Answer from the drawing. Dimensions are ordinates in mm from the lowest x, y and z of the part. A direction names the side the tool comes from. Coordinates: 2 decimals unless noted, no trailing zeros. Order: outer loops, then holes, each group sorted by start corner. A loop starts at its lowest first (then second) coordinate and runs counter-clockwise, first axis right, second up.
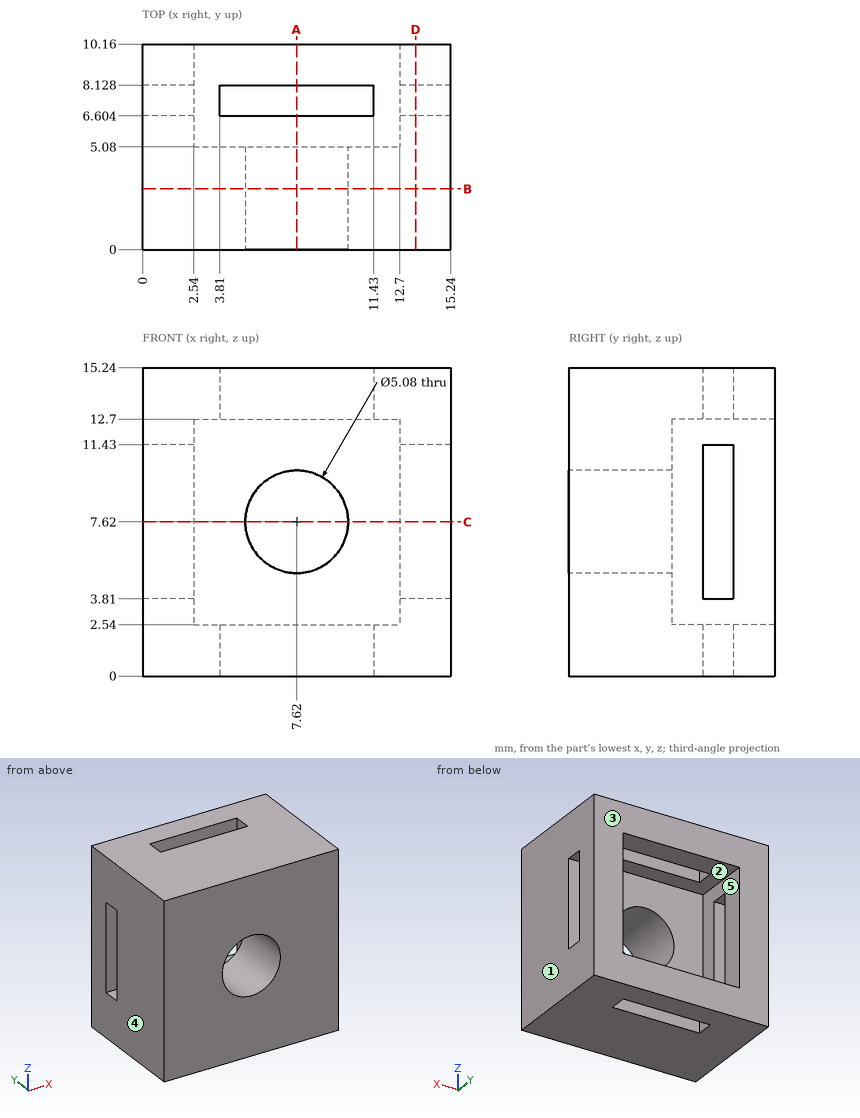
1) Section B-B (y = 3) is taken. Give the vertices of the cut face in (x, z), then the cut area to 3 significant figures.
2) Determine the mould class of the marked faces 1, 2 and 3 for opening direction X: released by +X, released by -X, zero draft, split by the parting line, or undercut.
3) Section A-A (x = 7.62) is taken. Give the vertices of the cut face in (y, z).
4) Consider L1, parallel to Z at x = 3.25, y = 7.5; L2, parallel to X at y = 3.2, z = 7.62. Determine where each line is inside the solid, lowest interval first.
5) Section D-D (x = 13.5) is taken. Give the vertices of the cut face in (y, z).
6) A tool of negligible diameter and unlimited length cuts with its end or side. For the marked faces 4 and 5, from which of +Z, -Z, +X, -X, +Y, -Y can it reach the whole face along a straight path? Write none if from no direction.
7) Section C-C (z = 7.62) is taken. Give the vertices of the cut face in (x, y).
Filled sheet:
1. outline: (0, 0) - (15.24, 0) - (15.24, 15.24) - (0, 15.24) - close; hole circle Ø5.08 at (7.62, 7.62)
1. area: 212 mm2
2. face 1: released by +X
2. face 2: undercut
2. face 3: zero draft
3. outline: (0, 0) - (6.6, 0) - (6.6, 2.54) - (5.08, 2.54) - (5.08, 5.08) - (0, 5.08) - close; (0, 10.16) - (5.08, 10.16) - (5.08, 12.7) - (6.6, 12.7) - (6.6, 15.24) - (0, 15.24) - close; (8.13, 0) - (10.16, 0) - (10.16, 2.54) - (8.13, 2.54) - close; (8.13, 12.7) - (10.16, 12.7) - (10.16, 15.24) - (8.13, 15.24) - close
4. L1: z = 0 to 2.54, 12.7 to 15.24
4. L2: x = 0 to 5.08, 10.16 to 15.24
5. outline: (0, 0) - (10.16, 0) - (10.16, 15.24) - (0, 15.24) - close; hole (6.6, 3.81) - (8.13, 3.81) - (8.13, 11.43) - (6.6, 11.43) - close
6. face 4: +Z, -Z, -X, +Y, -Y
6. face 5: +Y
7. outline: (0, 0) - (5.08, 0) - (5.08, 5.08) - (2.54, 5.08) - (2.54, 6.6) - (0, 6.6) - close; (0, 8.13) - (2.54, 8.13) - (2.54, 10.16) - (0, 10.16) - close; (10.16, 0) - (15.24, 0) - (15.24, 6.6) - (12.7, 6.6) - (12.7, 5.08) - (10.16, 5.08) - close; (12.7, 8.13) - (15.24, 8.13) - (15.24, 10.16) - (12.7, 10.16) - close
